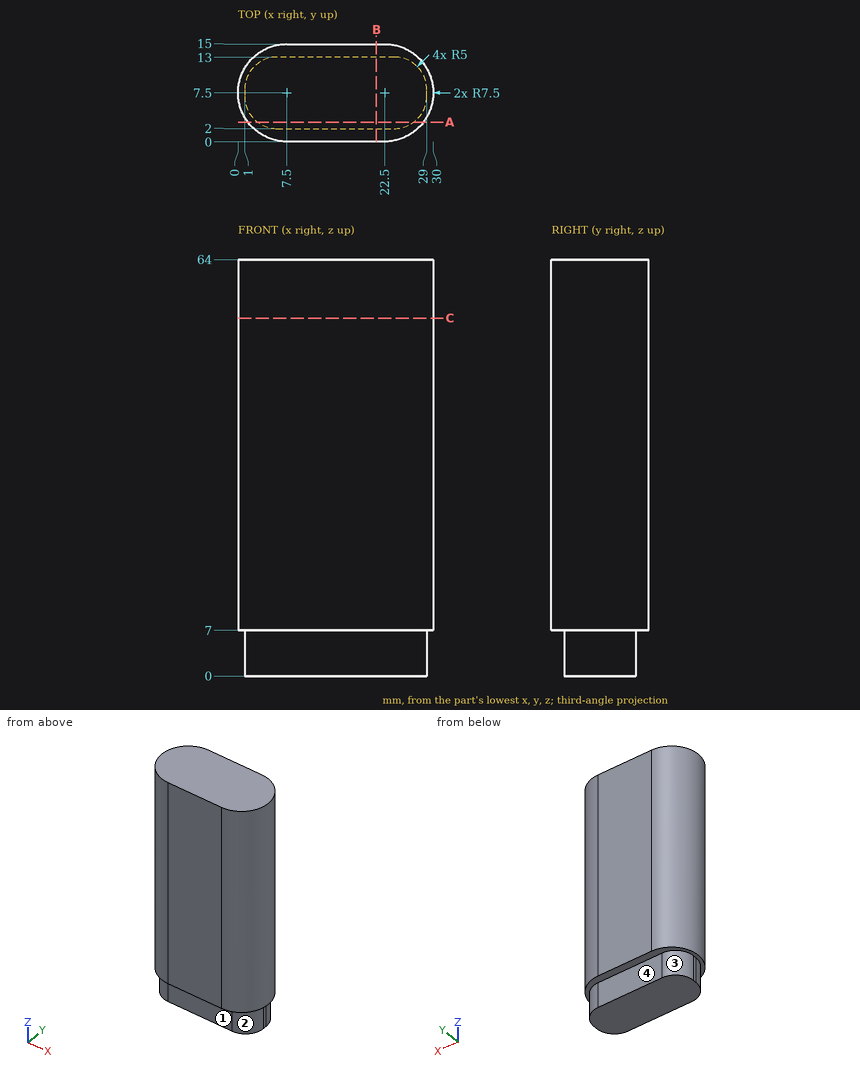
Print and shaded views of the part. All mm, measured from the part's lowest x, y and z. A direction names the side the tool comes from. Round coordinates to 2 decimals unless told otherwise and drop trailing zeros. Write each loop counter-clockwise with the first axis right and the second up, starting at its lowest first coordinate (ties: lowest second). Pieces come first, ordered by that corner, then holes. Notation, with made-up numbers: (12, 3) - (16, 3) arc R20 cw to (16, 7) - close; hole circle Ø7 at (35.25, 14). An arc over 180 degrees is marked (long way). One line per question, with ' | ' between items.
1. Drop flat-ended pins along their axis: pin 1 Ø1.1 at (y, z) = (7.5, 4) entering from +X; pin 2 Ø3 at (y, z) = (13, 7) entering from -X; pin 3 Ø1 at (x, z) = (6, 44) entering from +Y. Give the stop position or say it passes through.
Results are:
pin 1: x = 29 | pin 2: x = 1.16 | pin 3: y = 14.93
2. Band-saw the part on A-A, the plane y = 3. Write the cut outline in (x, z).
Results are:
outline: (1.5, 7) - (3, 7) - (3, 0) - (27, 0) - (27, 7) - (28.5, 7) - (28.5, 64) - (1.5, 64) - close
3. Band-saw the part on C-C, the plane z = 55. Write the cut outline in (x, y).
Results are:
outline: (7.5, 0) - (22.5, 0) arc R7.5 ccw to (22.5, 15) - (7.5, 15) arc R7.5 ccw to start
4. Drill centre lines: line 1 along Z through (x, y) = (7, 1.75); line 2 along X through (y, z) = (3.75, 61.5); line 3 along Y through (x, z) = (6.5, 38.5). Where is each one in solid material? Low to high. Write a range as from..to.
Results are:
line 1: 7..64 | line 2: 1..29 | line 3: 0.07..14.93
5. Band-saw the part on B-B, the plane x = 21.25. Write the cut outline in (y, z), and give its area (3 significant figures).
Results are:
outline: (0, 7) - (2, 7) - (2, 0) - (13, 0) - (13, 7) - (15, 7) - (15, 64) - (0, 64) - close | area: 932 mm^2
6. Tool access for the marked faces 1, 2, 3 and 4: list every direction of +Z, -Z, +X, -X, +Y, -Y with a clear straight run to the whole face (end or side of a thin tool).
Results are:
face 1: -Z, +X, -X, -Y | face 2: -Z, +X, -Y | face 3: -Z, -X, +Y | face 4: -Z, +X, -X, +Y
